CAD build for the part. Positions are in the model's coordinates, mm. Face numbers are marked on the shaded views. A direction names the side the tool comes from. Round coordinates to 2 decimals unless told otherwise and drop trailing zeros. Loops run counter-clockwise (first coordinate to the right, second up) from the corner with the lowest first, then second, coordinate; pieces in that order, holes last.
from build123d import *

# Parameters (mm, degrees)
BOSS_EXTRU_1_DEPTH      = 25
BOSS_EXTRU_1_DEPTH_BACK = 25
ESQUISSE1_R             = 22
BOSS_EXTRU_2_DEPTH      = 20.2
BOSS_EXTRU_2_DEPTH_BACK = 20.2
ESQUISSE5_R             = 15
ENL_V_MAT_EXTRU_1_DEPTH = 10.3
ESQUISSE7_R             = 12.75
ENL_V_MAT_EXTRU_3_DEPTH = 82.218329674
ESQUISSE8_R             = 10
ENL_V_MAT_EXTRU_4_DEPTH = 82.89474471
ESQUISSE9_R             = 18
ENL_V_MAT_EXTRU_5_DEPTH = 2
ENL_V_MAT_EXTRU_6_DEPTH = 82.218329674


with BuildPart() as part:
    # Esquisse1 → Boss.-Extru.1 (new, two sides: drawn at the far end of the back side and taken through both)
    with BuildSketch(Plane.XY.offset(-BOSS_EXTRU_1_DEPTH_BACK)):
        Circle(ESQUISSE1_R)
        with BuildLine():
            Line((-3, 9.539392014), (-3, 12.8))
            Line((-3, 12.8), (3, 12.8))
            Line((3, 12.8), (3, 9.539392014))
            ThreePointArc((3, 9.539392014), (8.062257748, 5.916079783), (10, 0))
            ThreePointArc((10, 0), (-5.916079783, -8.062257748), (-3, 9.539392014))
        make_face(mode=Mode.SUBTRACT)
    extrude(amount=BOSS_EXTRU_1_DEPTH + BOSS_EXTRU_1_DEPTH_BACK)

    # Esquisse4 → Boss.-Extru.2 (add, two sides: drawn at the far end of the back side and taken through both)
    with BuildSketch(Plane(origin=(0, 0, 0), x_dir=(0, 0, -1), z_dir=(1, 0, 0)).offset(-BOSS_EXTRU_2_DEPTH_BACK)):
        Polygon((1.045201898, -22), (-37.969134213, -61.014336111), (-49, -49.983470325), (-21.016529675, -22), (-21.016529675, 0), (0, 0), align=None)
    extrude(amount=BOSS_EXTRU_2_DEPTH + BOSS_EXTRU_2_DEPTH_BACK)

    # Esquisse5 → Enl_v. mat.-Extru.1 (cut)
    with BuildSketch(Plane(origin=(0, -0.491735162, -0.491735162), x_dir=(1, 0, 0), z_dir=(0, 0.7071067811865487, 0.7071067811865465))):
        with Locations(Location((0, -49.791883092, 0), (0, 0, 270))):
            Circle(ESQUISSE5_R)
    extrude(amount=-ENL_V_MAT_EXTRU_1_DEPTH, mode=Mode.SUBTRACT)

    # Esquisse7 → Enl_v. mat.-Extru.3 (cut, through all)
    with BuildSketch(Plane(origin=(0, -0.491735162, -0.491735162), x_dir=(1, 0, 0), z_dir=(0, 0.7071067811865487, 0.7071067811865465))):
        with Locations(Location((0, -49.791883092, 0), (0, 0, 270))):
            Circle(ESQUISSE7_R)
    extrude(amount=-ENL_V_MAT_EXTRU_3_DEPTH, mode=Mode.SUBTRACT)

    # Esquisse8 → Enl_v. mat.-Extru.4 (cut, through all)
    with BuildSketch(Plane.XY.offset(25)):
        Circle(ESQUISSE8_R)
    extrude(amount=-ENL_V_MAT_EXTRU_4_DEPTH, mode=Mode.SUBTRACT)

    # Esquisse9 → Enl_v. mat.-Extru.5 (cut)
    with BuildSketch(Plane(origin=(0, 0, -25), x_dir=(-1, 0, 0), z_dir=(0, 0, -1))):
        Circle(ESQUISSE9_R)
    extrude(amount=-ENL_V_MAT_EXTRU_5_DEPTH, mode=Mode.SUBTRACT)

    # Esquisse11 → Enl_v. mat.-Extru.6 (cut, through all)
    with BuildSketch(Plane(origin=(0, -0.491735162, -0.491735162), x_dir=(1, 0, 0), z_dir=(0, 0.7071067811865487, 0.7071067811865465))):
        with BuildLine():
            ThreePointArc((20.2, -50.204581464), (14.286537718, -64.07842081), (0.412698372, -69.991883092))
            Line((0.412698372, -69.991883092), (20.2, -69.991883092))
            Line((20.2, -69.991883092), (20.2, -50.204581464))
        make_face()
        with BuildLine():
            ThreePointArc((-0.412698372, -69.991883092), (-14.286537718, -64.07842081), (-20.2, -50.204581464))
            Line((-20.2, -50.204581464), (-20.2, -69.991883092))
            Line((-20.2, -69.991883092), (-0.412698372, -69.991883092))
        make_face()
    extrude(amount=-ENL_V_MAT_EXTRU_6_DEPTH, mode=Mode.SUBTRACT)


solid = part.part
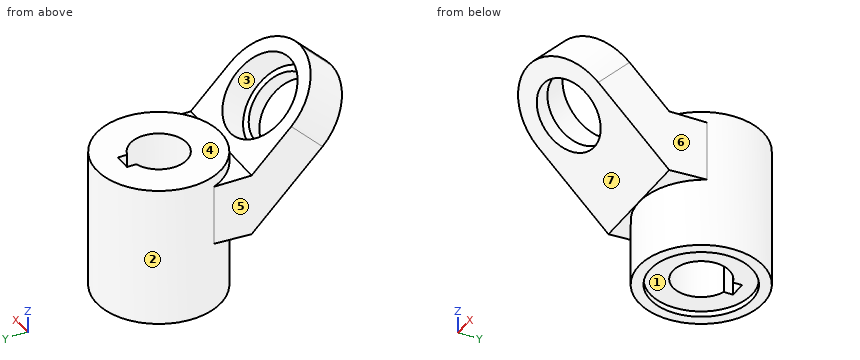
Item 1: Wall check: L1, parallel to Y at x = 0, z = -9.5; L2, parallel to Y at x = 0, z = -24; L3, parallel to Z at x = 9, y = -20. Give the ranges that are in metal, low to high.
Verdict:
L1: y = -22 to -10, 12.8 to 22
L2: y = -22 to -18, 18 to 22
L3: z = -25 to 25
Item 2: Cut at C-C (x = -4). List the corners of the cut face in (y, z).
Verdict:
outline: (-60.73, 37.69) - (-55.29, 32.25) - (-51.54, 35.99) - (-53.21, 37.66) - (-45.92, 44.94) - (-49.7, 48.72) - close; (-38.17, 15.13) - (-22, -1.05) - (-21.63, -1.03) - (-21.63, -25) - (-17.55, -25) - (-17.55, -23) - (-9.17, -23) - (-9.17, 25) - (-21.63, 25) - (-21.63, 21.02) - (-22, 21.02) - (-25.48, 24.49) - (-32.76, 17.21) - (-34.42, 18.87) - close; (9.17, -23) - (17.55, -23) - (17.55, -25) - (21.63, -25) - (21.63, 25) - (9.17, 25) - close
Item 3: Cut at A-A (y = 0). List the corners of the cut face in (x, z).
Verdict:
outline: (-22, -25) - (-18, -25) - (-18, -23) - (-10, -23) - (-10, 25) - (-22, 25) - close; (10, -23) - (18, -23) - (18, -25) - (22, -25) - (22, 25) - (10, 25) - close
Item 4: Flat gauge pins, fed straight in: P1, Ø3, axis at x = -1.5, z = 1, coming from the -Y side; P2, Ø6.5, axis at x = -5, y = -14, coming from the +Z side; P3, Ø4, axis at x = 13.5, y = -32.5, coming from the +Z side. Where does each tip first touch, or does it go through?
Verdict:
P1: stops at y = -25.55
P2: stops at z = 25
P3: stops at z = 33.03
Item 5: Cut at D-D (x = -11). List the corners of the cut face in (y, z), plus the area to 3 significant figures.
Verdict:
outline: (-58.71, 35.67) - (-51.29, 28.24) - (-47.54, 31.99) - (-50.19, 34.64) - (-42.91, 41.93) - (-47.68, 46.7) - close; (-42.17, 19.13) - (-22, -1.05) - (-19.05, -0.91) - (-19.05, -25) - (-14.25, -25) - (-14.25, -23) - (14.25, -23) - (14.25, -25) - (19.05, -25) - (19.05, 25) - (-19.05, 25) - (-19.05, 21.02) - (-22, 21.02) - (-28.49, 27.51) - (-35.77, 20.22) - (-38.42, 22.87) - close
area: 2,320 mm2
Item 6: Mould opens along X. For the marked faces 1, 2, 3 and 4 say: released by +X, released by -X, zero draft, split by the parting line, or undercut.
Verdict:
face 1: undercut
face 2: split by the parting line
face 3: undercut
face 4: zero draft
Item 7: 3-axis set-ups, long thin cutter, end or side, ignore diameter. For the marked faces 5, 6 and 7: which of +Z, -Z, +X, -X, +Y, -Y reach the whole face in a straight line?
Verdict:
face 5: +Z, -Z, -X, -Y
face 6: +Z, -Z, +X, -Y
face 7: -Z, +X, -X, -Y
Item 8: Cut at B-B (z = -5.5). List the corners of the cut face in (x, y).
Verdict:
outline: circle Ø44 at (0, 0); hole (-3, 9.54) arc R10 ccw (long way) to (3, 9.54) - (3, 12.8) - (-3, 12.8) - close
